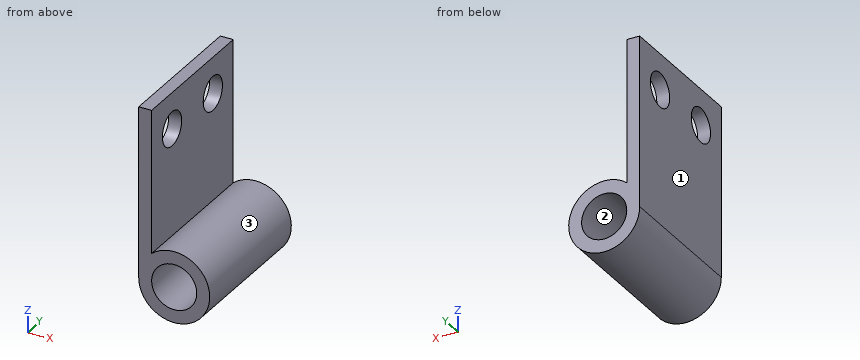
Autodesk Inventor part; units mm, degrees
ref_plane "YZ Plane" through (0, 0, 0) normal (1, 0, 0) x (0, 1, 0)
ref_plane "XZ Plane" through (0, 0, 0) normal (0, 1, 0) x (-1, 0, 0)
ref_plane "XY Plane" through (0, 0, 0) normal (0, 0, 1) x (1, 0, 0)
sketch "Sketch1" plane through (0, 0, 0) normal (0, 1, 0) x (-1, 0, 0)
  circle A0 centre (0, 0) radius 3.875
  circle A1 centre (0, 0) radius 4.375
  circle A2 centre (0, 0) radius 6.875
  line L0 (6.875, 0) -> (6.875, 33)
  line L1 (6.875, 33) -> (4.375, 33)
  line L2 (4.375, 33) -> (4.375, 5.3033)
  dimension "d0" = 7.75
  dimension "d1" = 8.75
  dimension "d2" = 13.75
  dimension "d3" = 33
  dimension "d4" = 2.5
extrude "Extrusion1" add sketch "Sketch1" along normal mid plane 28 contours A2 | A2 L2 L1 L0
sketch "Sketch4" plane through (-4.375, -14, 33) normal (1, 0, 0) x (0, 0, -1)
  line L0 (0, 28) -> (27.6967, 28)
  line L1 (0, 0) -> (0, 28)
  line L2 (0, 14) -> (27.6967, 14)
  line L3 (0, 14) -> (7, 14)
  line L4 (7, 14) -> (7, 7)
  line L5 (7, 14) -> (7, 21)
  point P0 (33, 14)
  dimension "d7" = 14
  dimension "d17" = 7
  dimension "d18" = 7
  dimension "d19" = 7
hole "Hole1" at (-4.375, -7, 26) at (-4.375, 7, 26) direction (-1, 0, 0) diameter 6.6 end up to surface
properties part number "SP29V1 Bisagra P1" material "Steel"
Model file for the job. Use its own axes, mm. Face numbers are marked on the shaded views. Give positions to 0.01 mm unless a question says otherwise; leave off trailing zeros. Order: outer loops, then holes, each group sorted by start corner. A loop starts at its lowest first (then second) coordinate and runs counter-clockwise, first axis right, second up. Notation, with made-up numbers: (11, 48.25) -> (55, 48.25) arc R27 ccw to (55, 85.25) -> close; hole circle Ø1 at (35, -19.75). An arc over 180 degrees is marked (long way). Use CSV: the item, a comma, the result in double quotes.
1. Band-saw the part on A-A, the plane y = -7. Give the cut face in (x, z) (3 decimals), then the cut area to 3 significant figures.
Outcome:
outline,"(-6.875, 0) arc R6.875 ccw (long way) to (-4.375, 5.303) -> (-4.375, 22.7) -> (-6.875, 22.7) -> close; (-6.875, 29.3) -> (-4.375, 29.3) -> (-4.375, 33) -> (-6.875, 33) -> close; hole circle Ø8.75 at (0, 0)"
area,"145 mm²"
2. Band-saw the part on B-B, the plane x = 0. Give the cut face in (y, z) (3 decimals).
Outcome:
outline,"(-14, -6.875) -> (14, -6.875) -> (14, -4.375) -> (-14, -4.375) -> close; (-14, 4.375) -> (14, 4.375) -> (14, 6.875) -> (-14, 6.875) -> close"
3. Band-saw the part on D-D, the plane z = -3. Give the cut face in (x, y).
Outcome:
outline,"(-6.19, -14) -> (-3.18, -14) -> (-3.18, 14) -> (-6.19, 14) -> close; (3.18, -14) -> (6.19, -14) -> (6.19, 14) -> (3.18, 14) -> close"
4. Band-saw the part on C-C, the plane z = 26. Give the cut face in (x, y) (3 decimals).
Outcome:
outline,"(-6.875, -14) -> (-4.375, -14) -> (-4.375, -10.3) -> (-6.875, -10.3) -> close; (-6.875, -3.7) -> (-4.375, -3.7) -> (-4.375, 3.7) -> (-6.875, 3.7) -> close; (-6.875, 10.3) -> (-4.375, 10.3) -> (-4.375, 14) -> (-6.875, 14) -> close"
5. Mould opens along Z. For the marked faces 1, 2 and 3 say: +Z half, -Z half, draft (parallel to the pull), parting line (faces both ways), or undercut.
Outcome:
face 1,"draft"
face 2,"undercut"
face 3,"parting line"
6. Drill centre lines: line 1 along Y through (x, z) = (-5.5, 26); line 2 along X through (y, z) = (0.25, 13.5) (3 decimals); line 3 along Z through (x, y) = (-1.5, 11.5). Where is each one in solid material? Low to high. Write a range as from..to.
Outcome:
line 1,"-14..-10.3, -3.7..3.7, 10.3..14"
line 2,"-6.875..-4.375"
line 3,"-6.71..-4.11, 4.11..6.71"
7. Drop flat-ended pins along their axis: pin 1 (7.5 mm diameter, centred on y = 7, z = 26, fed in from +X) (3 decimals); pin 2 (5 mm diameter, centred on x = 5, y = -4.5, fed in from +Z); pin 3 (6 mm diameter, centred on y = -7, z = 26, fed in from +X). Give the stop position or say it passes through.
Outcome:
pin 1,"x = -4.375"
pin 2,"z = 6.4"
pin 3,"through"
